Geometry check sheet. Reference: the model listing, model coordinates, mm. Face numbers are marked on the shaded views. A direction names the side the tool comes from. Coordinates: 2 decimals unless noted, no trailing zeros. Order: outer loops, then holes, each group sorted by start corner. A loop starts at its lowest first (then second) coordinate and runs counter-clockwise, first axis right, second up.
```python
from build123d import *

# Parameters (mm, degrees)
EXTRUDE_1_DEPTH     = 12
SKETCH_5_R          = 2.75
CUT_EXTRUDE_1_DEPTH = 35.132096332


with BuildPart() as part:
    # 草图1 → 凸台-拉伸1 (new, symmetric)
    with BuildSketch(Plane(origin=(0, 0, 0), x_dir=(1, 0, 0), z_dir=(0, 1, 0))):
        Polygon((5.5, 0), (-5.5, 0), (-5.5, 30), (-2.5, 30), (-2.5, 3), (2.5, 3), (2.5, 30), (5.5, 30), align=None)
    extrude(amount=EXTRUDE_1_DEPTH, both=True)

    # 草图5 → 切除-拉伸1 (cut, through all)
    with BuildSketch(Plane.ZY.offset(5.5)):
        with Locations((-10, 0)):
            Circle(SKETCH_5_R)
        with Locations((-19.5, 6)):
            Circle(SKETCH_5_R)
        with Locations((-19.5, -6)):
            Circle(SKETCH_5_R)
    extrude(amount=-CUT_EXTRUDE_1_DEPTH, mode=Mode.SUBTRACT)


solid = part.part
```
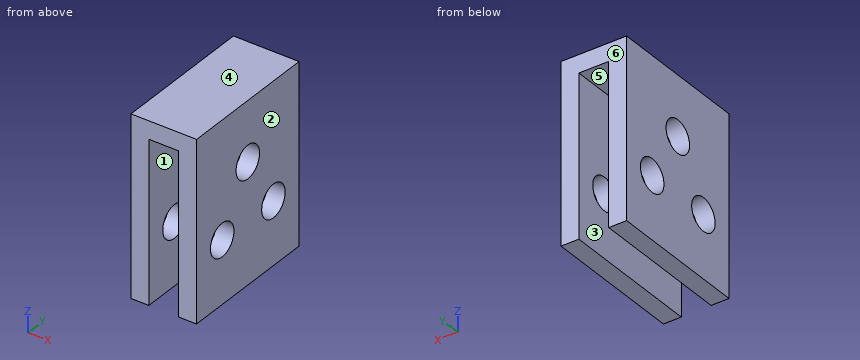
Item 1: Release check for a two-part mould opening along X. For the marked faces 1, 2, 3 and 4 record: pulls with the +X half, pulls with the -X half, needs draft (parallel to the pull), parting line crosses it, or undercut.
Item 2: Depth check by flat-ended pin: P1, Ø4.5, axis at y = 6, z = -19.5, coming from the -X side; P2, Ø2.5, axis at x = -0.5, y = -3.5, coming from the -Z side. Enter the tip coordinate at first touch or a pass-through.
Item 3: Thickness scan on line 1 along X through (y, z) = (0, -19.5); line 2 along Y through (x, z) = (3.25, -19.5); line 3 along Y through (x, z) = (-3.9, -10). Record the ranges inside material, lowest first.
Item 4: Sectioned sample at D-D (z = -15.5). Record the cut outline in (x, y), and give its area (3 significant figures).
Item 5: Tool access check on the marked faces 5 and 6. Record the directions out of +Z, -Z, +X, -X, +Y, -Y that give a thin tool (end or side, any length) a straight path to the whole face; none if there is none.
Item 6: Sectioned sample at C-C (x = 4). Record the cut outline in (y, z), and give its area (3 significant figures).
Item 7: Sectioned sample at B-B (y = -6). Record the cut outline in (x, z).
Item 8: Sectioned sample at A-A (z = -10). Record the cut outline in (x, y).
Geometry check:
1. face 1: undercut
1. face 2: pulls with the +X half
1. face 3: undercut
1. face 4: needs draft
2. P1: passes through
2. P2: stops at z = -3
3. line 1: x = -5.5 to -2.5, 2.5 to 5.5
3. line 2: y = -12 to -8.75, -3.25 to 3.25, 8.75 to 12
3. line 3: y = -12 to -2.75, 2.75 to 12
4. outline: (-5.5, -12) - (-2.5, -12) - (-2.5, 12) - (-5.5, 12) - close; (2.5, -12) - (5.5, -12) - (5.5, 12) - (2.5, 12) - close
4. area: 144 mm2
5. face 5: -Z, +Y, -Y
5. face 6: +Z, -Z, +X, -X, +Y
6. outline: (-12, -30) - (12, -30) - (12, 0) - (-12, 0) - close; hole circle Ø5.5 at (-6, -19.5); hole circle Ø5.5 at (0, -10); hole circle Ø5.5 at (6, -19.5)
6. area: 649 mm2
7. outline: (-5.5, -30) - (-2.5, -30) - (-2.5, -22.25) - (-5.5, -22.25) - close; (-5.5, -16.75) - (-2.5, -16.75) - (-2.5, -3) - (2.5, -3) - (2.5, -16.75) - (5.5, -16.75) - (5.5, 0) - (-5.5, 0) - close; (2.5, -30) - (5.5, -30) - (5.5, -22.25) - (2.5, -22.25) - close
8. outline: (-5.5, -12) - (-2.5, -12) - (-2.5, -2.75) - (-5.5, -2.75) - close; (-5.5, 2.75) - (-2.5, 2.75) - (-2.5, 12) - (-5.5, 12) - close; (2.5, -12) - (5.5, -12) - (5.5, -2.75) - (2.5, -2.75) - close; (2.5, 2.75) - (5.5, 2.75) - (5.5, 12) - (2.5, 12) - close
